```python
from build123d import *

# Parameters (mm, degrees)
ESQUISSE1_R        = 5.5
BOSS_EXTRU_1_DEPTH = 2
ESQUISSE2_R        = 2.4
ESQUISSE2_R_2      = 1.5
BOSS_EXTRU_2_DEPTH = 13
CONG_1_R           = 1


with BuildPart() as part:
    # Esquisse1 → Boss.-Extru.1 (new body)
    with BuildSketch(Plane.XY):
        Circle(ESQUISSE1_R)
    extrude(amount=BOSS_EXTRU_1_DEPTH)

    # Esquisse2 → Boss.-Extru.2 (add)
    with BuildSketch(Plane.XY.offset(2)):
        with Locations(Location((0, 0, 0), (0, 0, 180))):
            Circle(ESQUISSE2_R)
        with Locations(Location((0, 0, 0), (0, 0, 180))):
            Circle(ESQUISSE2_R_2, mode=Mode.SUBTRACT)
    extrude(amount=BOSS_EXTRU_2_DEPTH)

    # Congé1
    cong_1_edges = [part.edges().sort_by_distance(p)[0] for p in [
        (2.4, 0, 2),
    ]]
    fillet(cong_1_edges, radius=CONG_1_R)


solid = part.part
```
Design review of the part built by this model. Coordinates are the model's own, in mm. A direction names the side the tool comes from. Round coordinates to 2 decimals unless told otherwise and drop trailing zeros. Write each loop counter-clockwise with the first axis right and the second up, starting at its lowest first coordinate (ties: lowest second). Pieces come first, ordered by that corner, then holes. Notation, with made-up numbers: (79.5, -33) -> (94.5, -33) arc R4 cw to (94.5, -26) -> close; hole circle Ø3 at (66.5, 67.25). An arc over 180 degrees is marked (long way). Write item = value, one per line. Start each with the question number.
1) Wall thickness on probe 1 along Y at (x, z) = (0, 6.75); probe 2 along Z at (x, y) = (-2.75, 3.25); probe 3 along Y at (x, z) = (0.5, 4): over which ranges is each line inside the solid? List them lowest first. Write a range as from..to.
2) Take a section at D-D, the plane y = -4. State the section outline as (x, z) points, plus the area to 3 significant figures.
3) Take a section at C-C, the plane z = 6.75. State the section outline as (x, y) points, plus the area to 3 significant figures.
4) Tool access review of faces 1 (the face through (-1.29, -2.024, 8.916)), 2 (the face through (0, 2, 15)): name each direction out of +Z, -Z, +X, -X, +Y, -Y from which nothing blocks a thin tool from reaching the whole face with its end or side.
5) Mouldability with a two-part tool opening along X and no side actions: class faces 3 (the face through (0, 0, 0)), 4 (the face through (0, 0, 2)), 5 (the face through (-1.19, -5.37, 0.99)) as +X half, -X half, draft (parallel to the pull), parting line (faces both ways), or undercut.
6) Take a section at A-A, the plane x = 0. State the section outline as (y, z) points.
7) Clearance check with flat-ended pins moving along their axes: pin 1 (3 mm diameter, centred on y = -3.5, z = 2, fed in from -X); pin 2 (5 mm diameter, centred on x = 4, z = 6.5, fed in from +Y). State where each tip first meets the part, or that it passes through.
Results list:
q1.probe_1 = -2.4..-1.5, 1.5..2.4
q1.probe_2 = 0..2
q1.probe_3 = -2.35..-1.41, 1.41..2.35
q2.outline = (-3.77, 0) -> (3.77, 0) -> (3.77, 2) -> (-3.77, 2) -> close
q2.area = 15.1 mm²
q3.outline = circle Ø4.8 at (0, 0); hole circle Ø3 at (0, 0)
q3.area = 11.0 mm²
q4.face_1 = +Z
q4.face_2 = +Z, +X, -X, +Y, -Y
q5.face_3 = draft
q5.face_4 = undercut
q5.face_5 = parting line
q6.outline = (-5.5, 0) -> (5.5, 0) -> (5.5, 2) -> (3.4, 2) arc R1 cw to (2.4, 3) -> (2.4, 15) -> (1.5, 15) -> (1.5, 2) -> (-1.5, 2) -> (-1.5, 15) -> (-2.4, 15) -> (-2.4, 3) arc R1 cw to (-3.4, 2) -> (-5.5, 2) -> close
q7.pin_1 = -5.12
q7.pin_2 = 1.87
